Design review of the part built by this model. Coordinates are the model's own, in mm. A direction names the side the tool comes from. Coordinates: 2 decimals unless noted, no trailing zeros. Loops run counter-clockwise (first coordinate to the right, second up) from the corner with the lowest first, then second, coordinate; pieces in that order, holes last. Notation, with made-up numbers: (44, -33) -> (60, -33) arc R29 ccw to (60, -3) -> close; hole circle Ø4 at (84.5, -39.5). An arc over 180 degrees is marked (long way). Use a Markdown table: item, result. Add a question column.
Q1. Clearance check with flat-ended pins moving along their axes: pin 1 Ø6 at (y, z) = (13, 18.5) entering from +X; pin 2 Ø12.5 at (x, y) = (7.5, -7.5) entering from +Z; pin 3 Ø6 at (x, y) = (2.5, 10) entering from +Z; pin 4 Ø4 at (y, z) = (9, -29.5) entering from +X. State where each tip first meets the part, or that it passes through.
Q2. Take a section at A-A on x = 0. Write out the cut boundary in (y, z).
Q3. For faces 1 (the face through (20.03, 6.31, 8.87)), 2 (the face through (-4.8, -15.5, 0)), list the 3-axis set-ups (+Z, -Z, +X, -X, +Y, -Y) from which the entire face can be reached by the end or side of a thin tool; tool diameter is ignored.
Q4. Take a section at C-C on z = -13. Write out the cut boundary in (x, y).
Q5. Draft analysis for pull direction X (two halves, no side actions). For faces 3 (the face through (13.526, -7.648, 22.684)), 4 (the face through (-3.47, 15.62, -28.59)), 5 (the face through (-15, -7, 23)), 6 (the face through (0, 0, -58)), state which applies: pulls with the +X half, pulls with the -X half, needs draft (parallel to the pull), parting line crosses it, or undercut.
Q6. Take a section at D-D on y = -9. Write out the cut boundary in (x, z), plus the area to 3 significant figures.
Q7. For probe 1 along Z at (x, y) = (-15.5, -11.5); probe 2 along Z at (x, y) = (12, 2); probe 3 along Y at (x, z) = (0, -35.5), list the stretches that pass through material, from the lowest coordinate up.
from build123d import *

# Parameters (mm, degrees)
ESQUISSE1_R        = 21
BOSS_EXTRU_1_DEPTH = 18
ESQUISSE2_R        = 16
BOSS_EXTRU_2_DEPTH = 58
ESQUISSE7_R        = 2
BOSS_EXTRU_3_DEPTH = 9.5


with BuildPart() as part:
    # Esquisse1 → Boss.-Extru.1 (new body)
    with BuildSketch(Plane.XY):
        Circle(ESQUISSE1_R)
    extrude(amount=BOSS_EXTRU_1_DEPTH)

    # Esquisse2 → Boss.-Extru.2 (add)
    with BuildSketch(Plane(origin=(0, 0, 0), x_dir=(-1, 0, 0), z_dir=(0, 0, -1))):
        with Locations(Location((0, 0, 0), (0, 0, 180))):
            Circle(ESQUISSE2_R)
    extrude(amount=BOSS_EXTRU_2_DEPTH)

    # Esquisse7 → Boss.-Extru.3 (add)
    with BuildSketch(Plane.XY.offset(18)):
        with Locations((-15, -9)):
            Circle(ESQUISSE7_R)
        with Locations((15, -9)):
            Circle(ESQUISSE7_R)
    extrude(amount=BOSS_EXTRU_3_DEPTH)


solid = part.part
Answer list:
| question | item | result |
|---|---|---|
| 1 | pin 1 | x = 18.44 |
| 1 | pin 2 | z = 27.5 |
| 1 | pin 3 | z = 18 |
| 1 | pin 4 | x = 14.39 |
| 2 | outline | (-21, 0) -> (-16, 0) -> (-16, -58) -> (16, -58) -> (16, 0) -> (21, 0) -> (21, 18) -> (-21, 18) -> close |
| 3 | face 1 | +Z, -Z |
| 3 | face 2 | -Z |
| 4 | outline | circle Ø32 at (0, 0) |
| 5 | face 3 | undercut |
| 5 | face 4 | parting line crosses it |
| 5 | face 5 | undercut |
| 5 | face 6 | needs draft |
| 6 | outline | (-18.97, 0) -> (-13.23, 0) -> (-13.23, -58) -> (13.23, -58) -> (13.23, 0) -> (18.97, 0) -> (18.97, 18) -> (17, 18) -> (17, 27.5) -> (13, 27.5) -> (13, 18) -> (-13, 18) -> (-13, 27.5) -> (-17, 27.5) -> (-17, 18) -> (-18.97, 18) -> close |
| 6 | area | 2,290 mm² |
| 7 | probe 1 | 0 to 18 |
| 7 | probe 2 | -58 to 18 |
| 7 | probe 3 | -16 to 16 |
